```python
from build123d import *

# Parameters (mm, degrees)
F1_DEPTH  = 50
F2_R      = 10
F4_D      = 6
F5_R      = 3
F6_DEPTH  = 116.7873897197
F7_W      = 40
F7_H      = 34
F8_DEPTH  = 20
F9_W      = 40
F9_H      = 30
F10_DEPTH = 10
F11_R     = 10


with BuildPart() as f1:
    # F0 (on Right) → F1 (new body, symmetric)
    with BuildSketch(Plane.YZ):
        with BuildLine():
            Line((61.3908901802, 162.8224757301), (59.5115049387, 163.5065160167))
            Line((59.5115049387, 163.5065160167), (4.8845538596, 13.4202014333))
            ThreePointArc((4.8845538596, 13.4202014333), (6.0899596245, 4.2642356365), (14.2814800674, 0))
            Line((14.2814800674, 0), (124.2814800674, 0))
            Line((124.2814800674, 0), (124.2814800674, 2))
            Line((124.2814800674, 2), (14.2814800674, 2))
            ThreePointArc((14.2814800674, 2), (7.7282637131, 5.4113885092), (6.7639391011, 12.7361611466))
            Line((6.7639391011, 12.7361611466), (61.3908901802, 162.8224757301))
        make_face()
    extrude(amount=F1_DEPTH, both=True)

    # F2
    f2_edges = [f1.edges().sort_by_distance(p)[0] for p in [
        (-50, 60.451198, 163.164496),
        (50, 60.451198, 163.164496),
        (50, 124.28148, 1),
        (-50, 124.28148, 1),
    ]]
    fillet(f2_edges, radius=F2_R)

    # F4 (through all)
    with Locations(Plane(origin=(0, 0, 0), x_dir=(1, 0, 0), z_dir=(0, -0.9396926208, 0.3420201433))):
        with Locations((0, 125)):
            Hole(F4_D / 2)

    # F5 (on face) → F6 (cut, through all)
    with BuildSketch(Plane(origin=(0, 0, 0), x_dir=(1, 0, 0), z_dir=(0, -0.9396926208, 0.3420201433))):
        with Locations((-24, 134)):
            Circle(F5_R)
        with Locations((-24, 142)):
            Circle(F5_R)
        with Locations((-24, 150)):
            Circle(F5_R)
        with Locations((-24, 158)):
            Circle(F5_R)
        with Locations((-24, 166)):
            Circle(F5_R)
        with Locations((-16, 134)):
            Circle(F5_R)
        with Locations((-16, 142)):
            Circle(F5_R)
        with Locations((-16, 150)):
            Circle(F5_R)
        with Locations((-16, 158)):
            Circle(F5_R)
        with Locations((-16, 166)):
            Circle(F5_R)
        with Locations((-8, 134)):
            Circle(F5_R)
        with Locations((-8, 142)):
            Circle(F5_R)
        with Locations((-8, 150)):
            Circle(F5_R)
        with Locations((-8, 158)):
            Circle(F5_R)
        with Locations((-8, 166)):
            Circle(F5_R)
        with Locations((0, 134)):
            Circle(F5_R)
        with Locations((0, 142)):
            Circle(F5_R)
        with Locations((0, 150)):
            Circle(F5_R)
        with Locations((0, 158)):
            Circle(F5_R)
        with Locations((0, 166)):
            Circle(F5_R)
        with Locations((8, 134)):
            Circle(F5_R)
        with Locations((8, 142)):
            Circle(F5_R)
        with Locations((8, 150)):
            Circle(F5_R)
        with Locations((8, 158)):
            Circle(F5_R)
        with Locations((8, 166)):
            Circle(F5_R)
        with Locations((16, 134)):
            Circle(F5_R)
        with Locations((16, 142)):
            Circle(F5_R)
        with Locations((16, 150)):
            Circle(F5_R)
        with Locations((16, 158)):
            Circle(F5_R)
        with Locations((16, 166)):
            Circle(F5_R)
        with Locations((24, 134)):
            Circle(F5_R)
        with Locations((24, 142)):
            Circle(F5_R)
        with Locations((24, 150)):
            Circle(F5_R)
        with Locations((24, 158)):
            Circle(F5_R)
        with Locations((24, 166)):
            Circle(F5_R)
    extrude(amount=-F6_DEPTH, mode=Mode.SUBTRACT)

    # F7 (on face) → F8 (cut)
    with BuildSketch(Plane(origin=(0, 0, 0), x_dir=(1, 0, 0), z_dir=(0, -0.9396926208, 0.3420201433))):
        with Locations((0, 17)):
            Rectangle(F7_W, F7_H)
    extrude(amount=-F8_DEPTH, mode=Mode.SUBTRACT)

    # F9 (on face) → F10 (cut)
    with BuildSketch(Plane(origin=(0, 0, 0), x_dir=(1, 0, 0), z_dir=(0, 0, -1))):
        with Locations((0, -19.2814800674)):
            Rectangle(F9_W, F9_H)
    extrude(amount=-F10_DEPTH, mode=Mode.SUBTRACT)

    # F11
    f11_edges = [f1.edges().sort_by_distance(p)[0] for p in [
        (-20, 12.568377, 31.607529),
        (-20, 34.28148, 1),
        (20, 12.568377, 31.607529),
        (20, 34.28148, 1),
    ]]
    fillet(f11_edges, radius=F11_R)


solid = f1.part
```
Geometry check sheet. Reference: the model listing, model coordinates, mm. A direction names the side the tool comes from. Coordinates: 2 decimals unless noted, no trailing zeros. Order: outer loops, then holes, each group sorted by start corner. A loop starts at its lowest first (then second) coordinate and runs counter-clockwise, first axis right, second up.
Item 1: Mould release check, pull along X, two halves, no side actions. Record for faces 1 (the cylindrical face through (-34.79, 7.791, 5.324)), 2 (the flat face through (-50, 31, 83)), 3 (the cylindrical face through (-0.39, 53.25, 143.41)): released by +X, released by -X, zero draft, split by the parting line, or undercut.
Item 2: Section check D-D (x = -1). Count the separate pieces of the cut face and the enclosed holes in it, plus the area to 3 significant figures.
Item 3: Section check C-C (x = 38). Enter the section's corners in (y, z).
Item 4: Scan lines: line 1 along Z through (x, y) = (-40.5, 117); line 2 along Y through (x, z) = (-42, 58); line 3 along Y through (x, z) = (13, 98). Record each from-to range of solid material in increasing order.
Item 5: Tool access check on faces 4 (the cylindrical face through (9.38, 54.06, 145.63)), 5 (the flat face through (0.7, 33.695, 86.729)), 6 (the cylindrical face through (16.99, 31.43, 1.01)). Record the directions out of +Z, -Z, +X, -X, +Y, -Y that give a thin tool (end or side, any length) a straight path to the whole face; none if there is none.
Item 6: Depth check by flat-ended pin: pin 1 (6 mm diameter, centred on x = 29, z = 31, fed in from +Y); pin 2 (3 mm diameter, centred on x = 22.5, y = 104.5, fed in from +Z); pin 3 (12 mm diameter, centred on y = 22.5, z = 37.5, fed in from +X); pin 4 (2 mm diameter, centred on x = 5, z = 1, fed in from -Y). Enter the tip coordinate at first touch or a pass-through.
Item 7: Section check B-B (z = 16.5). Enter the section's corners in (x, y), plus the area to 3 significant figures.
Item 8: Section check A-A (x = -24). Enter the section's corners in (y, z), plus the area to 3 significant figures.
Check sheet entries:
1. face 1: zero draft
1. face 2: released by -X
1. face 3: undercut
2. separate pieces: 8
2. enclosed holes: 0
2. area: 392 mm2
3. outline: (4.88, 13.42) arc R10 ccw to (14.28, 0) - (124.28, 0) - (124.28, 2) - (14.28, 2) arc R8 cw to (6.76, 12.74) - (61.39, 162.82) - (59.51, 163.51) - close
4. line 1: z = 0 to 2
4. line 2: y = 21.11 to 23.24
4. line 3: y = 35.67 to 37.8
5. face 4: none
5. face 5: +X, -X, +Y
5. face 6: -Z, -Y
6. pin 1: stops at y = 14.5
6. pin 2: stops at z = 2
6. pin 3: passes through
6. pin 4: stops at y = 34.28
7. outline: (-50, 6.01) - (-20, 6.01) - (-20, 8.13) - (-50, 8.13) - close; (20, 6.01) - (50, 6.01) - (50, 8.13) - (20, 8.13) - close
7. area: 128 mm2
8. outline: (4.88, 13.42) arc R10 ccw to (14.28, 0) - (124.28, 0) - (124.28, 2) - (14.28, 2) arc R8 cw to (6.76, 12.74) - (46.68, 122.42) - (44.8, 123.1) - close; (46.86, 128.74) - (48.74, 128.05) - (49.42, 129.93) - (47.54, 130.62) - close; (49.59, 136.26) - (51.47, 135.57) - (52.16, 137.45) - (50.28, 138.13) - close; (52.33, 143.77) - (54.21, 143.09) - (54.89, 144.97) - (53.01, 145.65) - close; (55.07, 151.29) - (56.94, 150.61) - (57.63, 152.49) - (55.75, 153.17) - close; (57.8, 158.81) - (59.68, 158.12) - (61.39, 162.82) - (59.51, 163.51) - close
8. area: 514 mm2
